Here's how the part is built. I have some questions about the finished solid (model axes, mm). Round coordinates to 2 decimals unless told otherwise and drop trailing zeros. Order: outer loops, then holes, each group sorted by start corner. A loop starts at its lowest first (then second) coordinate and runs counter-clockwise, first axis right, second up. Notation, with made-up numbers: (9.25, -9.5) -> (27.25, -9.5) arc R19 cw to (27.25, 7.5) -> close; hole circle Ø11 at (-23, -34). An arc over 180 degrees is marked (long way). Use a Markdown table: item, result. Add a question column.
(1) I want a section at B-B, the plane z = 4. Please give me the cut outline in (x, y).
(2) I want a section at C-C, the plane y = 49. Please give me the cut outline in (x, z), then the cut area to 3 significant figures.
(3) I want a section at A-A, the plane x = 6. Please give me the cut outline in (y, z), then the cut area to 3 significant figures.
(4) I'm going to push flat-ended pins straight in: P1, Ø5, axis at y = 47.5, z = 4, coming from the -X side; P2, Ø5, axis at x = 30, y = 56, coming from the -Z side; P3, Ø1.5, axis at x = 50.5, y = 50.5, coming from the -Z side; P4, Ø6, axis at x = 13, y = 50, coming from the +Z side. Where does each tip first touch, or does it pass through?
(5) If I drill on probe 1 along Y at (x, z) = (57.5, 0.75); probe 2 along Y at (x, z) = (5, -5); probe 3 along Z at (x, y) = (53, 46), over which ranges is the centre line in solid material (lowest first)?
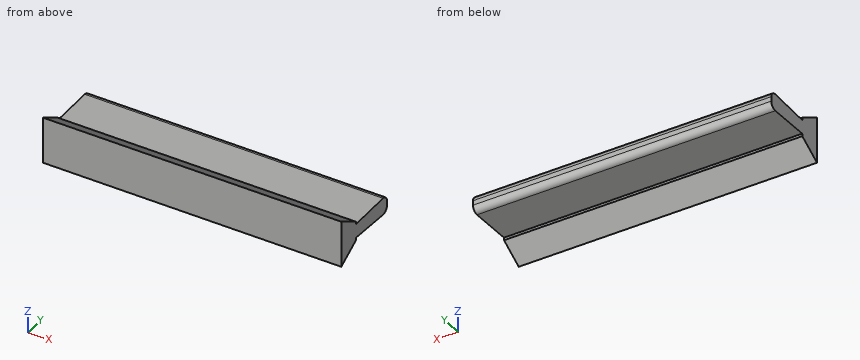
Autodesk Inventor part; units mm, degrees
ref_plane "YZ Plane" through (0, 0, 0) normal (1, 0, 0) x (0, 1, 0)
ref_plane "XZ Plane" through (0, 0, 0) normal (0, 1, 0) x (-1, 0, 0)
ref_plane "XY Plane" through (0, 0, 0) normal (0, 0, 1) x (1, 0, 0)
sketch "Sketch1" plane through (0, 0, 0) normal (1, 0, 0) x (0, 1, 0)
  arc A0 (63.4973, -0.5882) -> (63.4973, 0.5882) centre (0, 0) ccw
  line L0 (50.7691, -1.7729) -> (61.8544, -2.16)
  line L1 (50.7691, 1.7729) -> (61.8544, 2.16)
  arc A1 (63.4973, 0.5882) -> (61.8544, 2.16) centre (61.9098, 0.5735) ccw
  arc A2 (61.8544, -2.16) -> (63.4973, -0.5882) centre (61.9098, -0.5735) ccw
  arc A3 (2.7261, 50.7268) -> (-2.7261, 50.7268) centre (0, 0) ccw
  line L2 (44.704, 5.9101) -> (44.704, -5.9101)
  line L3 (44.704, 5.9101) -> (50.7421, 2.4239)
  line L4 (44.704, -5.9101) -> (50.7421, -2.4239)
  arc A4 (50.7421, -2.4239) -> (50.7691, -1.7729) centre (0, 0) ccw
  arc A5 (50.7691, 1.7729) -> (50.7421, 2.4239) centre (0, 0) ccw
  line L5 (63.5, 0) -> (73.7693, 0) construction
  point P0 (63.4613, -2.2161)
  point P1 (63.4613, 2.2161)
  point P2 (50.7268, -2.7261)
  dimension "d9" = 1.5875
extrude "Extrusion1" add sketch "Sketch1" along normal blind 76.2
properties part number "220525 Notch 0.5 inch"
Taken from the geometry:
| question | item | result |
|---|---|---|
| 1 | outline | (0, 44.7) -> (76.2, 44.7) -> (76.2, 48.01) -> (0, 48.01) -> close |
| 2 | outline | (0, -3.43) -> (76.2, -3.43) -> (76.2, 3.43) -> (0, 3.43) -> close |
| 2 | area | 523 mm2 |
| 3 | outline | (44.7, -5.91) -> (50.74, -2.42) arc R52.97 ccw to (50.77, -1.77) -> (61.85, -2.16) arc R1.59 ccw to (63.5, -0.59) arc R63.5 ccw to (63.5, 0.59) arc R1.59 ccw to (61.85, 2.16) -> (50.77, 1.77) arc R48.8 ccw to (50.74, 2.42) -> (44.7, 5.91) -> close |
| 3 | area | 100 mm2 |
| 4 | P1 | stops at x = 0 |
| 4 | P2 | stops at z = -2.04 |
| 4 | P3 | stops at z = -3 |
| 4 | P4 | stops at z = 4.58 |
| 5 | probe 1 | y = 44.7 to 63.49 |
| 5 | probe 2 | y = 44.7 to 46.28 |
| 5 | probe 3 | z = -5.16 to 5.16 |
